Read the model definition and answer for the solid it produces. Units are mm, in the model's axes. A direction names the side the tool comes from. Coordinates: 2 decimals unless noted, no trailing zeros. Write each loop counter-clockwise with the first axis right and the second up, starting at its lowest first coordinate (ties: lowest second). Pieces come first, ordered by that corner, then holes. Notation, with made-up numbers: M 53,-7 L 106,-7 A14 ccw 106,-2 Z; hole C -19.5,79 d7. An arc over 180 degrees is marked long. Write item = value, one per line.
from build123d import *

# Parameters (mm, degrees)
F0_W      = 102.108002
F0_H      = 126.492004
F1_DEPTH  = 75.946
F2_W      = 96.012
F2_H      = 120.700798
F3_DEPTH  = 67.818
F5_W      = 96.219298
F5_H      = 27.314827
F6_DEPTH  = 30.988
F7_W      = 97.910039
F7_H      = 17.801825
F8_DEPTH  = 25.4
F9_W      = 96.860379
F9_H      = 11.997812
F10_DEPTH = 25.4
F11_W     = 100.584
F11_H     = 4.876796
F12_DEPTH = 0.762


with BuildPart() as f1:
    # F0 (on Top) → F1 (new body)
    with BuildSketch(Plane.XY):
        with Locations((0.609599, -3.505202)):
            Rectangle(F0_W, F0_H)
    extrude(amount=-F1_DEPTH)

    # F2 (on face) → F3 (cut)
    with BuildSketch(Plane.XY):
        with Locations((0.9144, -3.047999)):
            Rectangle(F2_W, F2_H)
    extrude(amount=-F3_DEPTH, mode=Mode.SUBTRACT)

    # F5 (on face) → F6 (cut)
    with BuildSketch(Plane.XZ.offset(66.751204)):
        with Locations((0.171637, -13.657413)):
            Rectangle(F5_W, F5_H)
    extrude(amount=-F6_DEPTH, mode=Mode.SUBTRACT)

    # F7 (on face) → F8 (cut)
    with BuildSketch(Plane.XZ.offset(66.751204)):
        with Locations((0.818689, -45.399124)):
            Rectangle(F7_W, F7_H)
    extrude(amount=-F8_DEPTH, mode=Mode.SUBTRACT)

    # F9 (on face) → F10 (cut)
    with BuildSketch(Plane.XZ.offset(66.751204)):
        with Locations((1.082152, -68.534743)):
            Rectangle(F9_W, F9_H)
    extrude(amount=-F10_DEPTH, mode=Mode.SUBTRACT)

    # F11 (on Top) → F12 (join)
    with BuildSketch(Plane.XY):
        with Locations((1.3716, -64.617602)):
            Rectangle(F11_W, F11_H)
    extrude(amount=-F12_DEPTH)


solid = f1.part
Item 1: Flat-ended cylindrical pins translate along their axes: pin 1 (6 mm diameter, centred on x = 18, z = -71, fed in from -Y); pin 2 (8 mm diameter, centred on x = 34, y = 5, fed in from +Z); pin 3 (7.5 mm diameter, centred on x = -9, y = -52.5, fed in from +Z). Find the tip coordinate at first contact, or state that the pin passes through.
Worked answers:
pin_1 = -41.35
pin_2 = -67.82
pin_3 = -74.53
Item 2: Consider line 1 along X through (y, z) = (34, -47); line 2 along Y through (x, z) = (14, -30.5); line 3 along Z through (x, y) = (-28.5, 24.5). Determine where each line is inside the solid, lowest interval first. Write a range as from..to.
Worked answers:
line_1 = -50.44..-47.09, 48.92..51.66
line_2 = -66.75..-63.4, 57.3..59.74
line_3 = -75.95..-67.82
Item 3: Which of the six approach directions +Z, -Z, +X, -X, +Y, -Y give full straight-line access (tool end or side, diameter ignored) to faces 4 (the face through (49.774, -54, -46)), 5 (the face through (1, -63.398, -30)), 6 (the face through (51.664, -5, -37))?
Worked answers:
face_4 = -Y
face_5 = none
face_6 = +Z, -Z, +X, +Y, -Y
Item 4: Find section C-C (y = -57.5). Determine the outline of the cut face in (x, z), and give its area (3 significant figures).
Worked answers:
outline = M -50.44,-75.95 L 51.66,-75.95 L 51.66,0 L 48.92,0 L 48.92,-36.5 L 49.77,-36.5 L 49.77,-54.3 L 48.92,-54.3 L 48.92,-62.54 L 49.51,-62.54 L 49.51,-74.53 L -47.35,-74.53 L -47.35,-62.54 L -47.09,-62.54 L -47.09,-54.3 L -48.14,-54.3 L -48.14,-36.5 L -47.09,-36.5 L -47.09,-27.31 L -47.94,-27.31 L -47.94,0 L -50.44,0 Z
area = 531 mm²
Item 5: Find section B-B (x = -6.5). Determine the outline of the cut face in (y, z), and give its area (3 significant figures).
Worked answers:
outline = M -67.06,-0.76 L -62.18,-0.76 L -62.18,0 L -67.06,0 Z; M -66.75,-75.95 L 59.74,-75.95 L 59.74,0 L 57.3,0 L 57.3,-67.82 L -41.35,-67.82 L -41.35,-74.53 L -66.75,-74.53 Z; M -66.75,-62.54 L -63.4,-62.54 L -63.4,-54.3 L -66.75,-54.3 Z; M -66.75,-36.5 L -63.4,-36.5 L -63.4,-27.31 L -66.75,-27.31 Z
area = 1,090 mm²
Item 6: For a pull along X with two mould halves and no side action, classify faces 1 (the face through (0, 57.302, -33)), 2 (the face through (0, -3, -75.946)), 3 (the face through (-50.444, -4, -37)) as released by +X, released by -X, zero draft, split by the parting line, or undercut.
Worked answers:
face_1 = undercut
face_2 = zero draft
face_3 = released by -X
Item 7: Find section A-A (z = -61). Determine the outline of the cut face in (x, y), and give its area (3 significant figures).
Worked answers:
outline = M -50.44,-66.75 L 51.66,-66.75 L 51.66,59.74 L -50.44,59.74 Z; hole M -47.09,-63.4 L 48.92,-63.4 L 48.92,57.3 L -47.09,57.3 Z
area = 1,330 mm²
Item 8: Find section D-D (z = -49.5). Determine the outline of the cut face in (x, y), and give its area (3 significant figures).
Worked answers:
outline = M -50.44,-66.75 L -48.14,-66.75 L -48.14,-41.35 L -47.09,-41.35 L -47.09,57.3 L 48.92,57.3 L 48.92,-41.35 L 49.77,-41.35 L 49.77,-66.75 L 51.66,-66.75 L 51.66,59.74 L -50.44,59.74 Z
area = 957 mm²
